Answer from the drawing. Dimensions are ordinates in mm from the lowest x, y and z of the part. A direction names the side the tool comes from. Round coordinates to 2 decimals unless told otherwise and drop trailing zeros. Write each loop counter-clockwise with the first axis right and the second up, starting at its lowest first coordinate (ties: lowest second). Pieces come first, ordered by that corner, then holes.
1. Find section D-D (x = 174.5). Write down the section's boundary in (y, z).
2. Find section C-C (x = 66). Write down the section's boundary in (y, z).
3. A tool of negligible diameter and unlimited length cuts with its end or side. For the marked faces 1, 2 and 3, from which of +Z, -Z, +X, -X, +Y, -Y can it reach the whole face along a straight path? Write none if from no direction.
4. Flat-ended cylindrical pins translate along their axes: pin 1 Ø4 at (y, z) = (20.5, 17) entering from -X; pin 2 Ø8 at (x, y) = (154.5, 19.5) entering from +Z; pin 3 Ø2 at (x, y) = (105.5, 9.5) entering from +Z. Find the tip coordinate at first contact, or state that the pin passes through.
5. Find section A-A (y = 12.5). Write down the section's boundary in (x, z), and give its area (4 significant figures).
6. Straight lines are drawn through the part: probe 1 along X at (y, z) = (4.75, 8.5); probe 2 along Y at (x, z) = (159, 12); probe 3 along Z at (x, y) = (112.5, 5). For each, find the intervals that lie inside material, in ascending order.
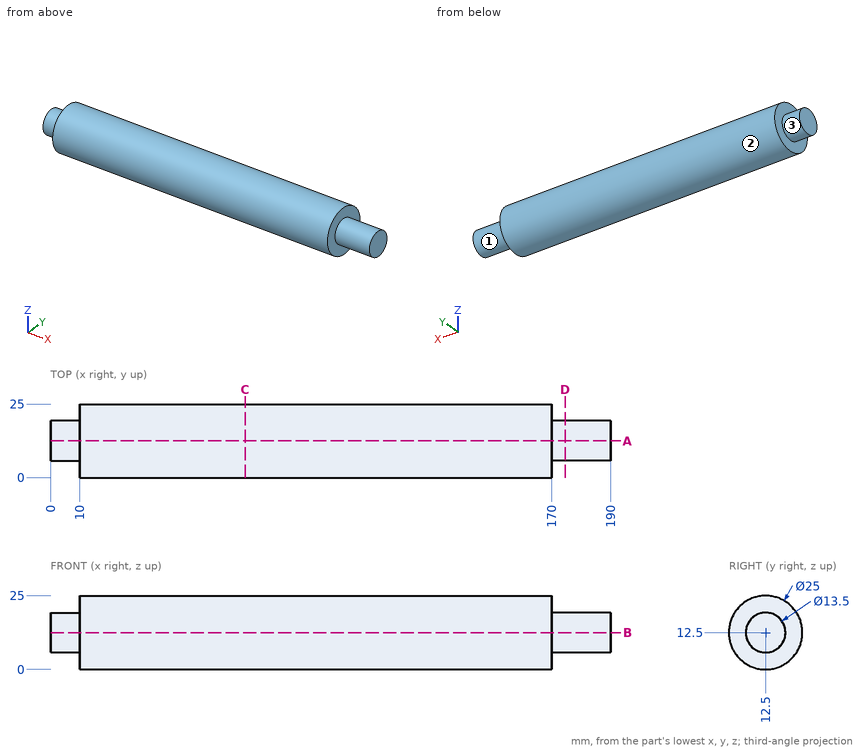
Worked answers:
1. outline: circle Ø13.5 at (12.5, 12.5)
2. outline: circle Ø25 at (12.5, 12.5)
3. face 1: +X
3. face 2: +X, -X
3. face 3: -X
4. pin 1: stops at x = 10
4. pin 2: stops at z = 24.63
4. pin 3: stops at z = 24.84
5. outline: (0, 5.75) - (10, 5.75) - (10, 0) - (170, 0) - (170, 5.75) - (190, 5.75) - (190, 19.25) - (170, 19.25) - (170, 25) - (10, 25) - (10, 19.25) - (0, 19.25) - close
5. area: 4,405 mm2
6. probe 1: x = 10 to 170
6. probe 2: y = 0.01 to 24.99
6. probe 3: z = 2.5 to 22.5
